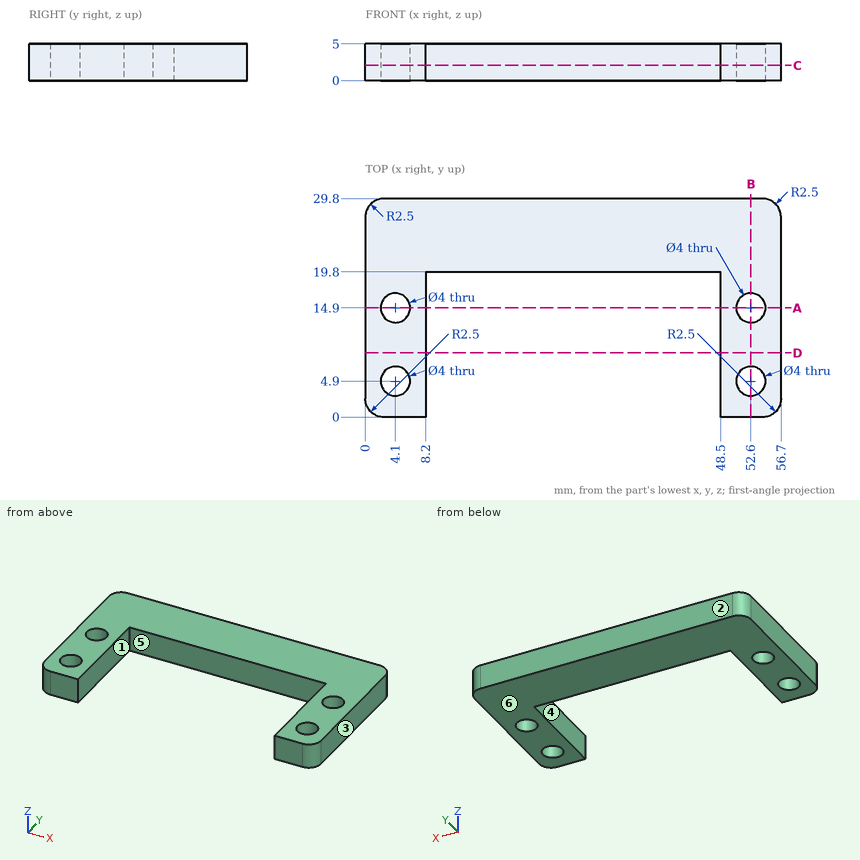
Print and shaded views of the part. All mm, measured from the part's lowest x, y and z. A direction names the side the tool comes from. Coordinates: 2 decimals unless noted, no trailing zeros. Order: outer loops, then holes, each group sorted by start corner. A loop starts at its lowest first (then second) coordinate and runs counter-clockwise, first axis right, second up. Notation, with made-up numbers: (64, -15) -> (119, -15) arc R27 ccw to (119, 5) -> close; hole circle Ø3 at (73.5, 46.5). An arc over 180 degrees is marked (long way). Answer as a JSON object with one key per item and string values. Group by question number.
1) Cut at A-A, the plane y = 14.9. Write the cut outline in (x, z), then the cut area to 3 significant figures.
2) Pull direction X, two halves, no side cores. Call the marked faces 3, 4, 5 and 6: +X half, -X half, draft (parallel to the pull), parting line (faces both ways), or undercut.
3) Drill centre lines: L1, parallel to Y at x = 52.6, z = 3.8; L2, parallel to X at y = 5, z = 3.55; L3, parallel to X at y = 8.5, z = 0.85. Where is each one in solid material? Low to high.
4) Which spindle directions (+Z, -Z, +X, -X, +Y, -Y) get a long thin tool onto all of the face, cutting with end or side? Do the marked faces 1 and 2. Say none if no direction does.
5) Flat gauge pins, fed straight in: pin 1 (1 mm diameter, centred on x = 31.5, z = 1.5, fed in from -Y); pin 2 (2.5 mm diameter, centred on x = 4.1, y = 14.9, fed in from +Z). Where does each tip first touch, or does it go through?
6) Cut at B-B, the plane x = 52.6. Write the cut outline in (y, z), then the cut area to 3 significant figures.
7) Cut at D-D, the plane y = 8.75. Write the cut outline in (x, z).
8) Cut at C-C, the plane z = 2.1. Write the cut outline in (x, y).
Check values:
{
 "1": {"outline": "(0, 0) -> (2.1, 0) -> (2.1, 5) -> (0, 5) -> close; (6.1, 0) -> (8.2, 0) -> (8.2, 5) -> (6.1, 5) -> close; (48.5, 0) -> (50.6, 0) -> (50.6, 5) -> (48.5, 5) -> close; (54.6, 0) -> (56.7, 0) -> (56.7, 5) -> (54.6, 5) -> close", "area": "42.0 mm²"},
 "2": {"face 3": "+X half", "face 4": "undercut", "face 5": "undercut", "face 6": "draft"},
 "3": {"L1": "y = 0 to 2.9, 6.9 to 12.9, 16.9 to 29.8", "L2": "x = 0 to 2.1, 6.1 to 8.2, 48.5 to 50.6, 54.6 to 56.7", "L3": "x = 0 to 8.2, 48.5 to 56.7"},
 "4": {"face 1": "+Z, -Z, -Y", "face 2": "+Z, -Z, +X, -X, +Y"},
 "5": {"pin 1": "stops at y = 19.8", "pin 2": "passes through"},
 "6": {"outline": "(0, 0) -> (2.9, 0) -> (2.9, 5) -> (0, 5) -> close; (6.9, 0) -> (12.9, 0) -> (12.9, 5) -> (6.9, 5) -> close; (16.9, 0) -> (29.8, 0) -> (29.8, 5) -> (16.9, 5) -> close", "area": "109 mm²"},
 "7": {"outline": "(0, 0) -> (8.2, 0) -> (8.2, 5) -> (0, 5) -> close; (48.5, 0) -> (56.7, 0) -> (56.7, 5) -> (48.5, 5) -> close"},
 "8": {"outline": "(0, 2.5) arc R2.5 ccw to (2.5, 0) -> (8.2, 0) -> (8.2, 19.8) -> (48.5, 19.8) -> (48.5, 0) -> (54.2, 0) arc R2.5 ccw to (56.7, 2.5) -> (56.7, 27.3) arc R2.5 ccw to (54.2, 29.8) -> (2.5, 29.8) arc R2.5 ccw to (0, 27.3) -> close; hole circle Ø4 at (4.1, 4.9); hole circle Ø4 at (4.1, 14.9); hole circle Ø4 at (52.6, 4.9); hole circle Ø4 at (52.6, 14.9)"}
}
